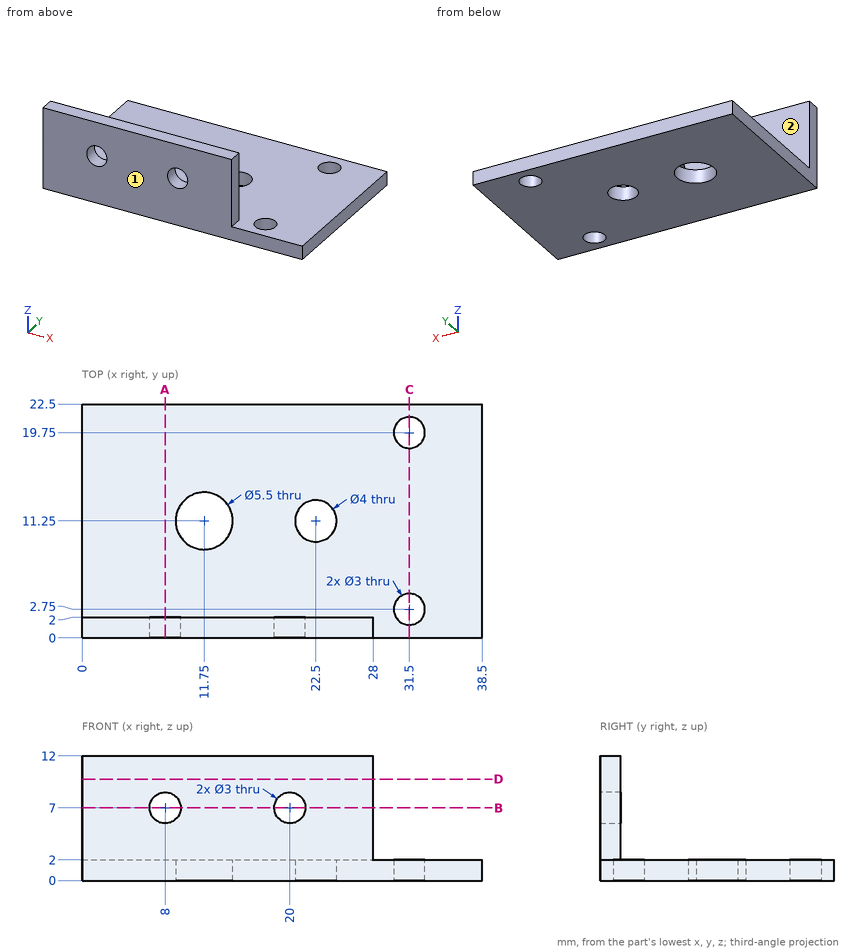
For this review, use the dimensioned drawing (mm, ordinates from the lowest corner) and the shaded views. A direction names the side the tool comes from. Give positions to 0.01 mm unless a question says otherwise; leave off trailing zeros. Write each loop counter-clockwise with the first axis right and the second up, starting at its lowest first coordinate (ties: lowest second). Pieces come first, ordered by that corner, then holes. Notation, with made-up numbers: M -27.75,13.5 L 31.25,13.5 A22 cw 31.25,41.5 Z; hole C 18,-12.75 d10. An arc over 180 degrees is marked long. Answer as a JSON object with one key per item and string values. Group by question number.
1) We need section D-D (z = 9.75). Give the boundary of the cut face in (x, y).
2) We need section A-A (x = 8). Give the boundary of the cut face in (y, z).
3) For line 1 along Y through (x, z) = (31.5, 1.55); line 2 along X through (y, z) = (0.55, 7); line 3 along Y through (x, z) = (9.5, 3), list the stretches that pass through material, from the lowest coordinate up.
4) We need section B-B (z = 7). Give the boundary of the cut face in (x, y), and give its area (3 significant figures).
5) We need section C-C (x = 31.5). Give the boundary of the cut face in (y, z), and give its area (3 significant figures).
6) Tool access review of the marked faces 1 and 2: name each direction out of +Z, -Z, +X, -X, +Y, -Y from which nothing blocks a thin tool from reaching the whole face with its end or side.
7) Clearance check with flat-ended pins moving along their axes: pin 1 Ø3 at (y, z) = (5, 7) entering from +X; pin 2 Ø1 at (y, z) = (1, 6) entering from +X; pin 3 Ø5 at (x, y) = (31.5, 2.75) entering from +Z; pin 4 Ø1 at (x, z) = (16, 5) entering from +Y. State where each tip first meets the part, or that it passes through.
Answer key:
{
 "1": {"outline": "M 0,0 L 28,0 L 28,2 L 0,2 Z"},
 "2": {"outline": "M 0,0 L 22.5,0 L 22.5,2 L 2,2 L 2,5.5 L 0,5.5 Z; M 0,8.5 L 2,8.5 L 2,12 L 0,12 Z"},
 "3": {"line 1": "y = 0 to 1.25, 4.25 to 18.25, 21.25 to 22.5", "line 2": "x = 0 to 6.5, 9.5 to 18.5, 21.5 to 28", "line 3": "y = 0 to 2"},
 "4": {"outline": "M 0,0 L 6.5,0 L 6.5,2 L 0,2 Z; M 9.5,0 L 18.5,0 L 18.5,2 L 9.5,2 Z; M 21.5,0 L 28,0 L 28,2 L 21.5,2 Z", "area": "44.0 mm²"},
 "5": {"outline": "M 0,0 L 1.25,0 L 1.25,2 L 0,2 Z; M 4.25,0 L 18.25,0 L 18.25,2 L 4.25,2 Z; M 21.25,0 L 22.5,0 L 22.5,2 L 21.25,2 Z", "area": "33.0 mm²"},
 "6": {"face 1": "+Z, -Z, +X, -X, -Y", "face 2": "+Z, +X, -X, +Y"},
 "7": {"pin 1": "passes through", "pin 2": "stops at x = 28", "pin 3": "stops at z = 2", "pin 4": "stops at y = 2"}
}
